Autodesk Inventor part; units mm, degrees
ref_plane "YZ Plane" through (0, 0, 0) normal (1, 0, 0) x (0, 1, 0)
ref_plane "XZ Plane" through (0, 0, 0) normal (0, 1, 0) x (-1, 0, 0)
ref_plane "XY Plane" through (0, 0, 0) normal (0, 0, 1) x (1, 0, 0)
sketch "Sketch1" plane through (0, 0, 0) normal (0, 1, 0) x (-1, 0, 0)
  line L0 (0, 0) -> (0, -111.226) construction
  line L1 (-3, 0) -> (-3, -111.226)
  line L2 (3, -111.226) -> (3, 0)
  arc A0 (3, 0) -> (-3, 0) centre (0, 0) ccw
  arc A1 (-3, -111.226) -> (3, -111.226) centre (0, -111.226) ccw
  circle A2 centre (0, 0) radius 1.5
  circle A3 centre (0, -111.226) radius 1.5
  arc A4 (3, 0) -> (3, -111.226) centre (399.1151, -55.613) ccw
  arc A5 (-3, 0) -> (-3, -111.226) centre (393.1151, -55.613) ccw
  point P0 (0, -55.613)
  dimension "d0" = 111.226
  dimension "d1" = 6
  dimension "d2" = 3
  dimension "d3" = 3
  dimension "d10" = 400
  dimension "d11" = 400
extrude "Extrusion1" add sketch "Sketch1" along normal blind 8 contours A0 A4 A1 L1 | L1 A5
sketch "Sketch2" plane through (0, 0, 0) normal (0, -1, 0) x (1, 0, 0)
  arc A0 (3, 0) -> (-3, 0) centre (0, 0) ccw
  arc A1 (-3, -111.226) -> (-3, 0) centre (-399.1151, -55.613) ccw
  arc A2 (-3, -111.226) -> (3, -111.226) centre (0, -111.226) ccw
  arc A3 (3, -111.226) -> (3, 0) centre (-393.1151, -55.613) ccw
  circle A4 centre (0, -111.226) radius 1.5
  circle A5 centre (0, 0) radius 1.5
The model under review builds one solid part; all positions refer to its coordinate system, in mm. Give positions to 0.01 mm unless a question says otherwise; leave off trailing zeros. Write each loop counter-clockwise with the first axis right and the second up, starting at its lowest first coordinate (ties: lowest second). Pieces come first, ordered by that corner, then holes.
1. For P1, Ø3, axis at y = 1, z = -34.5, coming from the +X side; P2, Ø1.8, axis at x = 0, z = -111.226, coming from the +Y side; P3, Ø4, axis at y = 3, z = -39, coming from the +X side; P4, Ø1, axis at y = 5.5, z = -100, coming from the -X side, all flat-tipped, find the tip position at first contact; note any pin that passes through.
2. Add section B-B, the plane z = -6. Write out the cut boundary in (x, y), plus the area to 3 significant figures.
3. Wall thickness on L1, parallel to X at y = 6.5, z = -52.5; L2, parallel to X at y = 4.25, z = -83: over which ranges is each line inside the solid? List them lowest first.
4. Add section A-A, the plane y = 5. Write out the cut boundary in (x, z).
5. Draft analysis for pull direction Z (two halves, no side actions). For faces 1 (the cylindrical face through (-0.066, 3.944, -114.225)), 2 (the cylindrical face through (1.5, 3.94, -0.07)), 3 (the cylindrical face through (6.884, 3.944, -56.394)), 4 (the cylindrical face through (0.884, 3.944, -56.394)), state which applies: +Z half, -Z half, draft (parallel to the pull), parting line (faces both ways), or undercut.
Worked answers:
1. P1: stops at x = 6.4
1. P2: passes through
1. P3: stops at x = 6.62
1. P4: stops at x = -1.64
2. outline: (-2.2, 0) - (3.8, 0) - (3.8, 8) - (-2.2, 8) - close
2. area: 48.0 mm2
3. L1: x = 0.87 to 6.87
3. L2: x = -0.05 to 5.95
4. outline: (-3, -111.23) arc R3 ccw to (3, -111.23) arc R400 ccw to (3, 0) arc R3 ccw to (-3, 0) arc R400 cw to start; hole circle Ø3 at (0, -111.23); hole circle Ø3 at (0, 0)
5. face 1: -Z half
5. face 2: undercut
5. face 3: parting line
5. face 4: undercut
